Here's how the part is built. I have some questions about the finished solid (model axes, mm). A direction names the side the tool comes from. Give positions to 0.01 mm unless a question says otherwise; leave off trailing zeros. Order: outer loops, then holes, each group sorted by start corner. A loop starts at its lowest first (then second) coordinate and runs counter-clockwise, first axis right, second up.
from build123d import *

# Parameters (mm, degrees)
CYLINDER_R     = 48
CYLINDER_DEPTH = 43
BOX001_W       = 50
BOX001_H       = 140
BOX001_DEPTH   = 20
BOX002_W       = 55
BOX002_H       = 100
BOX002_DEPTH   = 20
BOX003_W       = 28
BOX003_H       = 36
BOX003_DEPTH   = 20
BOX004_W       = 40
BOX004_H       = 40
BOX004_DEPTH   = 10
BOX_W          = 300
BOX_H          = 300
BOX_DEPTH      = 13


with BuildPart() as cylinder:
    # Cylinder → Cylinder (new body)
    with BuildSketch(Plane(origin=(150, 150, 13), x_dir=(1, 0, 0), z_dir=(0, 0, 1))):
        Circle(CYLINDER_R)
    extrude(amount=CYLINDER_DEPTH)


with BuildPart() as battery:
    # Box001 → Box001 (new body)
    with BuildSketch(Plane(origin=(20, 70, 13), x_dir=(1, 0, 0), z_dir=(0, 0, 1))):
        with Locations((25, 70)):
            Rectangle(BOX001_W, BOX001_H)
    extrude(amount=BOX001_DEPTH)


with BuildPart() as arduino:
    # Box002 → Box002 (new body)
    with BuildSketch(Plane(origin=(240, 10, 13), x_dir=(1, 0, 0), z_dir=(0, 0, 1))):
        with Locations((27.5, 50)):
            Rectangle(BOX002_W, BOX002_H)
    extrude(amount=BOX002_DEPTH)


with BuildPart() as maestro:
    # Box003 → Box003 (new body)
    with BuildSketch(Plane(origin=(136, 10, 13), x_dir=(1, 0, 0), z_dir=(0, 0, 1))):
        with Locations((14, 18)):
            Rectangle(BOX003_W, BOX003_H)
    extrude(amount=BOX003_DEPTH)


with BuildPart() as obj1:
    # Box004 → Box004 (new body)
    with BuildSketch(Plane(origin=(170, 60, 13), x_dir=(1, 0, 0), z_dir=(0, 0, 1))):
        with Locations((20, 20)):
            Rectangle(BOX004_W, BOX004_H)
    extrude(amount=BOX004_DEPTH)


with BuildPart() as base:
    # Box → Box (new body)
    with BuildSketch(Plane.XY):
        with Locations((150, 150)):
            Rectangle(BOX_W, BOX_H)
    extrude(amount=BOX_DEPTH)

    # Fusion: union Cylinder, Battery, Arduino, Maestro, obj1
    add(cylinder.part)
    add(battery.part)
    add(arduino.part)
    add(maestro.part)
    add(obj1.part)


solid = base.part
Q1. If we section it at C-C on x = 150: List the corners of the cut face in (y, z) for me.
Filled sheet:
outline: (0, 0) - (300, 0) - (300, 13) - (198, 13) - (198, 56) - (102, 56) - (102, 13) - (46, 13) - (46, 33) - (10, 33) - (10, 13) - (0, 13) - close
Q2. I'm going to push flat-ended pins straight in: P1, Ø10, axis at x = 257.5, z = 19.5, coming from the -Y side; P2, Ø22, axis at y = 44, z = 27.5, coming from the -X side; P3, Ø12, axis at x = 153.5, z = 38, coming from the +Y side. Where does each tip first touch, or does it pass through?
Filled sheet:
P1: stops at y = 10
P2: stops at x = 136
P3: stops at y = 198
Q3. If we section it at A-A on x = 61: List the corners of the cut face in (y, z) for me, plus the area to 3 significant figures.
Filled sheet:
outline: (0, 0) - (300, 0) - (300, 13) - (210, 13) - (210, 33) - (70, 33) - (70, 13) - (0, 13) - close
area: 6,700 mm2
Q4. For faces 1 (the face through (267, 10, 23)), 2 (the face through (194.34, 131.62, 34.2)), 3 (the face through (170, 80, 18)), which set-ups out of +Z, -Z, +X, -X, +Y, -Y let a thin tool reach every point of the face, with its end or its side?
Filled sheet:
face 1: +Z, +X, -X, -Y
face 2: +Z
face 3: +Z, -Y
Q5. I need wall thicknesses on L1, parallel to Y at x = 42, z = 16; L2, parallel to Z at x = 110, y = 215; L3, parallel to Z at x = 161.5, y = 37. Which ranges of each line are inside material? Lowest first, please.
Filled sheet:
L1: y = 70 to 210
L2: z = 0 to 13
L3: z = 0 to 33
Q6. Thinking about a two-plate mould opening in X: for faces 4 (the face through (45, 70, 23)), 5 (the face through (300, 148, 6)), 6 (the face through (70, 139, 23)), which applies, released by +X, released by -X, zero draft, split by the parting line, or undercut?
Filled sheet:
face 4: zero draft
face 5: released by +X
face 6: undercut
Q7. If we section it at D-D on y = 263.5: List the corners of the cut face in (x, z) for me.
Filled sheet:
outline: (0, 0) - (300, 0) - (300, 13) - (0, 13) - close
Q8. If we section it at B-B on y = 150: List the corners of the cut face in (x, z) for me.
Filled sheet:
outline: (0, 0) - (300, 0) - (300, 13) - (198, 13) - (198, 56) - (102, 56) - (102, 13) - (70, 13) - (70, 33) - (20, 33) - (20, 13) - (0, 13) - close
